Input: part model. Units: mm. Frame: model coordinates. A direction names the side the tool comes from. Coordinates: 2 decimals unless noted, no trailing zeros. Order: outer loops, then holes, each group sorted by start corner. A loop starts at its lowest first (then second) coordinate and runs counter-clockwise, first axis right, second up. Notation, with made-up numbers: (18.5, 63.5) - (76.5, 63.5) arc R20 ccw to (76.5, 87.5) - close; hole circle Ø2 at (-35, 65). An arc over 180 degrees is marked (long way). Answer as CSV lines item,"result". Start each with the question number.
Item 1: Material intervals for line 1 along X through (y, z) = (2.7, -42); line 2 along X through (y, z) = (1.3, 0); line 3 along Z through (x, y) = (-30.5, 0.95), sorted ascending.
Item 2: Access query for faces 1 (the flat face through (5, 2, -27)), 2 (the cylindrical face through (16.5, 2.37, 0.07)), 3 (the flat face through (-20, 1.8, 12)), 4 (the flat face through (-28, 1, -35.633)), 5 (the cylindrical face through (-58.8, 2.43, -44.49)). Directions: +Z, -Z, +X, -X, +Y, -Y. A direction counts if a zero-diameter tool reaches every point of the face in a straight line with its end or side. Return the directions, or none.
Item 3: Draft query along X for faces 6 (the flat face through (-20, 1, 9.167)), 7 (the cylindrical face through (-9.5, 2.37, 0.07)), 8 (the flat face through (-60, 2, -13)), 9 (the flat face through (21.1, 2, 7)). Return one class per face: +X half, -X half, draft (parallel to the pull), parting line (faces both ways), or undercut.
Item 4: First-contact query: pin 1 (1.4 mm diameter, centred on x = -13.5, z = 11.5, fed in from -Y); pin 2 (2.5 mm diameter, centred on y = 1.5, z = -32.5, fed in from +X); pin 3 (2.5 mm diameter, centred on x = -40, z = -42, fed in from -Y). Flat tips, straight axial feed; report the tip coordinate or a pass-through.
Item 5: Section A-A (x = 0). Output: boundary loops of the cut face in (y, z), and give its area (3 significant figures).
Item 6: Section D-D (z = -32). Output: boundary loops of the cut face in (x, y), and give its area (3 significant figures).
Item 7: Section B-B (x = -19). Output: boundary loops of the cut face in (y, z).
Item 8: Section C-C (z = -16.5). Output: boundary loops of the cut face in (x, y).
Autodesk Fusion 360 part; units mm, degrees
sketch "Sketch1" plane through (0, 0, 0) normal (0, 1, 0) x (1, 0, 0)
  circle A0 centre (0, 0) radius 48 construction
  circle A1 centre (0, 0) radius 14 construction
  circle A2 centre (0, 0) radius 9.5 construction
  circle A3 centre (0, 0) radius 8 construction
  line L0 (0, 0) -> (8, 0) construction
  line L1 (0, 0) -> (0, -9.5) construction
  line L2 (0, 0) -> (-8, 0) construction
  line L3 (0, 0) -> (0, 9.5) construction
  circle A4 centre (8, 0) radius 1.5
  circle A5 centre (-8, 0) radius 1.5
  circle A6 centre (0, 9.5) radius 1.5
  circle A7 centre (0, 0) radius 12 construction
  line L4 (8, 0) -> (18, 0) construction
  line L5 (21.1, 0) -> (19.55, 2.6847) construction
  line L6 (19.55, 2.6847) -> (16.45, 2.6847) construction
  line L7 (16.45, 2.6847) -> (14.9, 0) construction
  line L8 (14.9, 0) -> (16.45, -2.6847) construction
  line L9 (16.45, -2.6847) -> (19.55, -2.6847) construction
  line L10 (19.55, -2.6847) -> (21.1, 0) construction
  circle A8 centre (18, 0) radius 3.1 construction
  circle A9 centre (18, 0) radius 1.5
  line L11 (0, 52) -> (-68, 52) construction
  line L12 (-9.7468, 47) -> (-68, 47) construction
  line L13 (-68, 52) -> (-68, 47) construction
  line L14 (-68, 47) -> (-68, 35.633) construction
  line L15 (-68, 35.633) -> (-32.1604, 35.633) construction
  line L16 (-68, 35.633) -> (-68, 30.833) construction
  line L17 (-68, 30.833) -> (-36.7876, 30.833) construction
  line L18 (-68, 30.833) -> (-68, -9.167) construction
  line L19 (-60, -9.167) -> (-47.1165, -9.167)
  line L20 (-68, -9.167) -> (-68, -13.967) construction
  line L21 (-68, -13.967) -> (-45.923, -13.967) construction
  line L22 (-60, -13.967) -> (-60, 35.633)
  line L23 (5.9333, 10.4305) -> (19.5328, 2.6945)
  line L24 (-60, -13.967) -> (21.1, -13.967)
  line L25 (21.1, -13.967) -> (21.1, 0)
  arc A10 (21.1, 0) -> (19.5328, 2.6945) centre (18, 0) ccw
  line L26 (-60, 35.633) -> (5, 35.633)
  line L27 (5, 35.633) -> (5, 11.8322)
  arc A11 (5.9333, 10.4305) -> (5.7778, 10.5175) centre (0, 0) ccw
  arc A12 (5, 11.8322) -> (5.7778, 10.5175) centre (6.5, 11.8322) ccw
  arc A13 (5.7778, 10.5175) -> (7.9656, 11.513) centre (6.5, 11.8322) ccw construction
  arc A14 (5.4445, 12.898) -> (5, 11.8322) centre (6.5, 11.8322) ccw construction
  arc A15 (7.9656, 11.513) -> (5.4445, 12.898) centre (6.5, 11.8322) ccw construction
  line L28 (5, 11.8322) -> (5, 10.9087) construction
  arc A16 (5.7778, 10.5175) -> (5, 10.9087) centre (0, 0) ccw construction
  line L29 (-60, 30.833) -> (5, 30.833)
  line L30 (-47.1165, -9.167) -> (21.1, -9.167)
  line L31 (-60, 35.633) -> (-60, 45.633)
  line L32 (-60, 45.633) -> (5, 45.633)
  line L33 (5, 45.633) -> (5, 35.633)
  circle A17 centre (-56, 42) radius 1.5
  circle A18 centre (-40, 42) radius 1.5
  line L34 (-40, 42) -> (0, 0) construction
  circle A19 centre (-55.8448, -4.167) radius 1.5
  line L35 (0, 0) -> (-55.8448, -4.167) construction
  line L36 (-68, -9.167) -> (-60, -9.167) construction
  point P0 (18, 0)
  point P1 (-33.1034, 34.7586)
  point P2 (-47.8669, -3.5717)
  dimension "d1" = 96
  dimension "d2" = 28
  dimension "d3" = 19
  dimension "d4" = 16
  dimension "d5" = 3
  dimension "d6" = 3
  dimension "d7" = 3
  dimension "d8" = 24
  dimension "d9" = 18
  dimension "d10" = 3.1
  dimension "d11" = 60
  dimension "d12" = 3
  dimension "d13" = 52
  dimension "d14" = 68
  dimension "d15" = 68
  dimension "d18" = 5
  dimension "d22" = 16.367
  dimension "d23" = 4.8
  dimension "d24" = 40
  dimension "d25" = 4.8
  dimension "d26" = 8
  dimension "d27" = 3.1
  dimension "d28" = 5
  dimension "d33" = 12
  dimension "d34" = 3
  dimension "d35" = 10
  dimension "d36" = 3
  dimension "d37" = 12
  dimension "d38" = 5
  dimension "d39" = 3
  dimension "d40" = 5
  dimension "d41" = 10
  dimension "d42" = 3
  dimension "d43" = 5
  dimension "d44" = 8
extrude "Extrude1" add sketch "Sketch1" along normal blind 4.8
fillet "Fillet1" radius 4 2 edges at (5, 2.4, -45.633) (-60, 2.4, -45.633)
extrude "Extrude2" cut sketch "Sketch1" along normal blind 1.8 contours L19 L22 L24 L25 L30 | L22 L26 L27 L29
Determined:
1,line 1,"x = -59.98 to -57.5, -54.5 to -41.5, -38.5 to 4.98"
1,line 2,"x = -60 to -9.5, -6.5 to 6.5, 9.5 to 16.5, 19.5 to 21.1"
1,line 3,"z = -45.63 to -35.63, -30.83 to 9.17"
2,face 1,"-Z, +X, +Y, -Y"
2,face 2,"+Y, -Y"
2,face 3,"+Z, +X, -X, -Y"
2,face 4,"+X, -X, -Y"
2,face 5,"-Z, -X, +Y, -Y"
3,face 6,"draft"
3,face 7,"undercut"
3,face 8,"-X half"
3,face 9,"+X half"
4,pin 1,"stops at y = 1.8"
4,pin 2,"stops at x = 5"
4,pin 3,"passes through"
5,outline,"(0, -45.63) - (4.8, -45.63) - (4.8, -11) - (0, -11) - (0, -30.83) - (1.8, -30.83) - (1.8, -35.63) - (0, -35.63) - close; (0, -8) - (4.8, -8) - (4.8, 13.97) - (1.8, 13.97) - (1.8, 9.17) - (0, 9.17) - close"
5,area,"254 mm^2"
6,outline,"(-60, 1.8) - (5, 1.8) - (5, 4.8) - (-60, 4.8) - close"
6,area,"195 mm^2"
7,outline,"(0, -45.63) - (4.8, -45.63) - (4.8, 13.97) - (1.8, 13.97) - (1.8, 9.17) - (0, 9.17) - (0, -30.83) - (1.8, -30.83) - (1.8, -35.63) - (0, -35.63) - close"
8,outline,"(-60, 0) - (5, 0) - (5, 4.8) - (-60, 4.8) - close"
